```python
from build123d import *

# Parameters (mm, degrees)
THICKEN1_T2         = 2
SKETCH2_R           = 35
SKETCH2_R_2         = 33
BOSS_EXTRUDE1_DEPTH = 140


with BuildPart() as body_1:
    # Surface-Revolve1: a surface, the sketch's curves turned about an axis
    with BuildLine(Plane(origin=(0, 0, 0), x_dir=(1, 0, 0), z_dir=(0, 1, 0)), mode=Mode.PRIVATE) as surface_revolve1_1_path:
        Line((0, 0), (0, 15))
        ThreePointArc((0, 15), (5.857864376, 29.142135624), (20, 35))
    surface_revolve1_1 = Shell.revolve(surface_revolve1_1_path.wire(), 360, Axis((0, 0, 0), (1, 0, 0)))
    add(Solid.thicken(surface_revolve1_1, -THICKEN1_T2))

    # Sketch2 → Boss-Extrude1 (add)
    with BuildSketch(Plane(origin=(20, 0, 0), x_dir=(0, 0, -1), z_dir=(1, 0, 0))):
        Circle(SKETCH2_R)
        Circle(SKETCH2_R_2, mode=Mode.SUBTRACT)
    extrude(amount=BOSS_EXTRUDE1_DEPTH)


solid = body_1.part
```
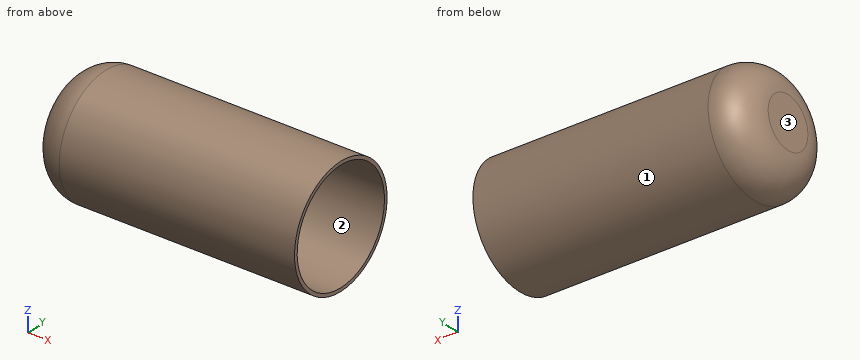
Part model, mm, in its own coordinate system. Face numbers are marked on the shaded views. Round coordinates to 2 decimals unless told otherwise and drop trailing zeros. Loops run counter-clockwise (first coordinate to the right, second up) from the corner with the lowest first, then second, coordinate; pieces in that order, holes last.
1. Drill centre lines: line 1 along Z through (x, y) = (130.5, 1); line 2 along Y through (x, z) = (126, 0); line 3 along Y through (x, z) = (82, -5). Where is each one in solid material? Low to high.
Solutions:
line 1: z = -34.99 to -32.98, 32.98 to 34.99
line 2: y = -35 to -33, 33 to 35
line 3: y = -34.64 to -32.62, 32.62 to 34.64
2. Two-plate mould, pull along Z, no slides. Class the marked faces 1, 2 and 3: pulls with the +Z half, pulls with the -Z half, needs draft (parallel to the pull), parting line crosses it, or undercut.
Solutions:
face 1: parting line crosses it
face 2: undercut
face 3: needs draft
3. Slice it at A-A (x = 45.5). Give the cut face in (y, z), and give its area (3 significant figures).
Solutions:
outline: circle Ø70 at (0, 0); hole circle Ø66 at (0, 0)
area: 427 mm2
4. Flat gauge pins, fed straight in: pin 1 (4 mm diameter, centred on x = 37, z = 1, fed in from +Y); pin 2 (8 mm diameter, centred on x = 103.5, y = 6, fed in from +Z); pin 3 (3 mm diameter, centred on y = 9, z = -14.5, fed in from +X); pin 4 (8 mm diameter, centred on x = 35, y = -0.5, fed in from -Z). Where does each tip first touch, or does it go through?
Solutions:
pin 1: stops at y = 35
pin 2: stops at z = 34.94
pin 3: stops at x = 2.36
pin 4: stops at z = -35
